Could you check a few things on this model? Use its own coordinates, in mm. A direction names the side the tool comes from. Coordinates: 2 decimals unless noted, no trailing zeros. Order: outer loops, then holes, each group sorted by start corner. A loop starts at its lowest first (then second) coordinate and runs counter-clockwise, first axis right, second up. Notation, with made-up numbers: (27.25, -23) -> (82.25, -23) arc R13 ccw to (82.25, -11) -> close; hole circle Ø9 at (9, 5.25). An arc over 180 degrees is marked (long way). Put each result on its own line as item: value. Start each with the question number.
Q1. If we section it at A-A (x = 103): Please give me the cut outline in (y, z), and give its area (3 significant figures).
Q2. We'd pull the mould along Z, two halves only. Please class faces 4 (the face through (125.4, 9, 9)), 5 (the face through (17.3, -0.73, -0.95)), 6 (the face through (-6, 0, -11)): +Z half, -Z half, draft (parallel to the pull), parting line (faces both ways), or undercut.
Q3. Please list where these lines run through material, in increasing order: line 1 along Y through (x, z) = (8.5, 0); line 2 along X through (y, z) = (3.5, 15).
Q4. For faces 1 (the face through (2.7, 0.3, 6.91)), 2 (the face through (-6, 0, 11)), 3 (the face through (-9.87, -12.38, -0.19)), which set-ups out of +Z, -Z, +X, -X, +Y, -Y let a thin tool reach every point of the face, with its end or its side?
Q5. If we section it at C-C (y = -18): Please give me the cut outline in (x, z), and give its area (3 significant figures).
Q6. If we section it at B-B (z = -20.5): Please give me the cut outline in (x, y), and give its area (3 significant figures).
Q7. Will these pins go through, and if not, where does the flat tip stop? pin 1 (4 mm diameter, centred on x = 47.5, z = 6.5, fed in from -Y); pin 2 (10 mm diameter, centred on x = 29.5, y = 21, fed in from +Z); pin 3 (4 mm diameter, centred on x = -5.5, y = 3, fed in from -Z); pin 4 (11 mm diameter, centred on y = 0, z = 0, fed in from -X).
from build123d import *

# Parameters (mm, degrees)
CUT_EXTRUDE_1_DEPTH       = 22
CUT_EXTRUDE_1_DEPTH_BACK  = 22
HOLE_WIZARD_1_D           = 13.835
HOLE_WIZARD_1_DEPTH       = 24
HOLE_WIZARD_1_CSINK_D     = 16
HOLE_WIZARD_1_CSINK_ANGLE = 90
HOLE_WIZARD_1_TIP         = 3.993820487


with BuildPart() as part:
    # Sketch 1 → Revolve 1 (revolve)
    with BuildSketch(Plane.XY, mode=Mode.PRIVATE) as revolve_1_sk:
        Polygon((-10, 0), (-10, 12.25), (-9.75, 12.5), (0, 12.5), (0, 0), align=None)
    revolve(revolve_1_sk.sketch.rotate(Axis((0, 0, 0), (-1, 0, 0)), 270), axis=Axis((0, 0, 0), (-1, 0, 0)))

    # Sketch 2 → Revolve 2 (revolve)
    with BuildSketch(Plane.XY, mode=Mode.PRIVATE) as revolve_2_sk:
        Polygon((0, 0), (0, 12.5), (125.4, 12.5), (125.4, 39.8), (142.5, 39.8), (142.5, 0), align=None)
    revolve(revolve_2_sk.sketch.rotate(Axis((142.5, 0, 0), (-1, 0, 0)), 270), axis=Axis((142.5, 0, 0), (-1, 0, 0)))

    # Sketch 3 → Cut-Extrude 1 (cut, two sides: drawn at the far end of the back side and taken through both)
    with BuildSketch(Plane(origin=(0, 0, 0), x_dir=(1, 0, 0), z_dir=(0, 1, 0)).offset(-CUT_EXTRUDE_1_DEPTH_BACK)):
        Polygon((-20, -16), (3.5, -16), (-1.5, -11), (-10, -11), (-10, 11), (-1.5, 11), (3.5, 16), (-20, 16), align=None)
    extrude(amount=CUT_EXTRUDE_1_DEPTH + CUT_EXTRUDE_1_DEPTH_BACK, mode=Mode.SUBTRACT)

    # Hole Wizard 1
    with Locations(Plane.ZY.offset(10)):
        with Locations((0, 0)):
            CounterSinkHole(HOLE_WIZARD_1_D / 2, HOLE_WIZARD_1_CSINK_D / 2, depth=HOLE_WIZARD_1_DEPTH, counter_sink_angle=HOLE_WIZARD_1_CSINK_ANGLE)
            with Locations((0, 0, -(HOLE_WIZARD_1_DEPTH + HOLE_WIZARD_1_TIP / 2))):  # 120° drill point
                Cone(0, HOLE_WIZARD_1_D / 2, HOLE_WIZARD_1_TIP, mode=Mode.SUBTRACT)


solid = part.part
The answers:
1. outline: circle Ø25 at (0, 0)
1. area: 491 mm^2
2. face 4: draft
2. face 5: undercut
2. face 6: -Z half
3. line 1: -12.5 to -6.92, 6.92 to 12.5
3. line 2: 125.4 to 142.5
4. face 1: -X
4. face 2: +Z, -X, +Y, -Y
4. face 3: -X, -Y
5. outline: (125.4, -35.5) -> (142.5, -35.5) -> (142.5, 35.5) -> (125.4, 35.5) -> close
5. area: 1,210 mm^2
6. outline: (125.4, -34.11) -> (142.5, -34.11) -> (142.5, 34.11) -> (125.4, 34.11) -> close
6. area: 1,170 mm^2
7. pin 1: y = -11.66
7. pin 2: through
7. pin 3: z = -11
7. pin 4: x = 14.82
